Geometry check sheet. Reference: the model listing, model coordinates, mm. A direction names the side the tool comes from. Round coordinates to 2 decimals unless told otherwise and drop trailing zeros. Order: outer loops, then holes, each group sorted by start corner. A loop starts at its lowest first (then second) coordinate and runs counter-clockwise, first axis right, second up. Notation, with made-up numbers: (15.5, 33) - (44.5, 33) arc R19 cw to (44.5, 45) - close; hole circle Ø5 at (30, 79.25). An arc over 180 degrees is marked (long way). Use a Markdown table: item, result. Add a question column.
(1) Thickness scan on line 1 along Z through (x, y) = (55.5, -24); line 2 along X through (y, z) = (-26.5, 6); line 3 along Y through (x, z) = (30.5, 9). Record the ranges inside material, lowest first. Write a range as [from, to].
(2) Gauge pin test, flat ends, axial feed: P1, Ø9.5, axis at y = -32.5, z = 20, coming from the +X side (3 decimals); P2, Ø9.5, axis at x = 45, y = -26.5, coming from the +Z side; P3, Ø1.5, axis at x = 28, z = 6.5, coming from the -Y side. Record the tip position at first contact, or that the pin passes through.
(3) Section check A-A on x = 28. Record the boundary of the cut face in (y, z).
(4) Section check B-B on y = -28. Record the boundary of the cut face in (x, z), then the cut area to 3 significant figures.
(5) Access from +Z, -Z, +X, -X, +Y, -Y to the whole of each face (thin tool, end or side, straight path). Record for faces 1 (the face through (-0.135, -28, 16)), 2 (the face through (-1, 0, 0)).
```python
from build123d import *

# Parameters (mm, degrees)
F0_W     = 127
F0_H     = 63.5
F1_DEPTH = 38.1
F3_DEPTH = 60.96


with BuildPart() as f1:
    # F0 (on Front) → F1 (new body)
    with BuildSketch(Plane.XZ):
        Rectangle(F0_W, F0_H)
    extrude(amount=F1_DEPTH)

    # F2 (on Top) → F3 (cut)
    with BuildSketch(Plane.XY):
        Polygon((-0.134974, -19.093526), (-0.134974, -35.547902), (-0.134974, -38.143526), (63.365026, -38.143526), (74.700989, -38.143526), (74.700989, -19.093526), (63.365026, -19.093526), align=None)
    extrude(amount=F3_DEPTH, mode=Mode.SUBTRACT)


solid = f1.part
```
Check sheet entries:
| question | item | result |
|---|---|---|
| 1 | line 1 | z = [-31.75, 0] |
| 1 | line 2 | x = [-63.5, -0.13] |
| 1 | line 3 | y = [-19.09, 0] |
| 2 | P1 | stops at x = -0.135 |
| 2 | P2 | stops at z = 0 |
| 2 | P3 | stops at y = -19.09 |
| 3 | outline | (-38.1, -31.75) - (0, -31.75) - (0, 31.75) - (-19.09, 31.75) - (-19.09, 0) - (-38.1, 0) - close |
| 4 | outline | (-63.5, -31.75) - (63.5, -31.75) - (63.5, 0) - (-0.13, 0) - (-0.13, 31.75) - (-63.5, 31.75) - close |
| 4 | area | 6,040 mm2 |
| 5 | face 1 | +Z, +X, -Y |
| 5 | face 2 | +Z, -Z, +X, -X, +Y |
